The listing builds one solid part. Answer for the finished solid, in the listing's coordinates (mm). A direction names the side the tool comes from. Coordinates: 2 decimals unless noted, no trailing zeros. Write each loop counter-clockwise with the first axis right and the second up, starting at its lowest first coordinate (ties: lowest second). Pieces come first, ordered by that corner, then holes.
(1) Straight lines are drawn through the part: line 1 (Z direction, x = -22, y = 50) (3 decimals); line 2 (X direction, y = 52.5, z = 26) (3 decimals); line 3 (Z direction, x = -67, y = 2) (3 decimals). For each, find the intervals that lie inside material, in ascending order.
(2) The part is cut by section B-B on x = 67.31. Determine the outline of the cut face in (y, z) (1 decimal), plus the area to 3 significant figures.
(3) The part is cut by section D-D on x = 32. Determine the outline of the cut face in (y, z) (3 decimals), plus the area to 3 significant figures.
(4) Given P1, Ø13.5, axis at x = -72, z = 75.5, coming from the +Y side (3 decimals); P2, Ø3, axis at x = -9, y = 51, coming from the -Z side; P3, Ø7.5, axis at x = 67.31, z = -79.375, coming from the -Y side; P4, Ø2, axis at x = -41, z = -2.5, coming from the -Y side (3 decimals), each flat-ended and moving along its own axis, determine where each tip first touches the part or whether it passes through.
(5) Which of the six approach directions +Z, -Z, +X, -X, +Y, -Y give full straight-line access (tool end or side, diameter ignored) to faces 1 (the flat face through (65, 3.175, -84)), 2 (the flat face through (-83.185, 40, 1)), 3 (the flat face through (48.26, 7, -79)), 4 (the flat face through (51.435, 12, 73))?
(6) The part is cut by section C-C on z = 3. Determine the outline of the cut face in (x, y) (3 decimals), plus the area to 3 significant figures.
(7) For a pull along X with two mould halves and no side action, classify faces 5 (the flat face through (84.813, 13.568, 83.599)), 6 (the flat face through (-65, 3.175, -84)) as +X half, -X half, draft (parallel to the pull), parting line (faces both ways), or undercut.
(8) The part is cut by section A-A on y = 31. Determine the outline of the cut face in (x, z) (3 decimals).
from build123d import *

# Parameters (mm, degrees)
SKETCH1_W                    = 172.72
SKETCH1_H                    = 127
BOSS_EXTRUDE1_DEPTH          = 83.82
SHELL1_T                     = -3.175
SKETCH6_W                    = 38.1
SKETCH6_H                    = 38.1
BOSS_EXTRUDE4_DEPTH          = 3.175
BOSS_EXTRUDE5_DEPTH          = 3.175
MIRROR5_COPY_1_DEPTH         = 3.175
MIRROR6_COPY_1_DEPTH         = 3.175
MIRROR6_COPY_2_SKETCH_W      = 38.1
MIRROR6_COPY_2_SKETCH_H      = 38.1
MIRROR6_COPY_2_DEPTH         = 3.175
MIRROR6_COPY_3_DEPTH         = 3.175
MIRROR6_COPY_4_DEPTH         = 3.175
FILLET3_R                    = 2.54
F_3_8_0_375_DIAMETER_HOLE1_D = 9.525
MIRROR8_COPY_1_D             = 9.525
FILLET4_R                    = 3.175


with BuildPart() as part:
    # Sketch1 → Boss-Extrude1 (new body)
    with BuildSketch(Plane(origin=(0, 0, 0), x_dir=(1, 0, 0), z_dir=(0, 1, 0))):
        Rectangle(SKETCH1_W, SKETCH1_H)
    extrude(amount=BOSS_EXTRUDE1_DEPTH)

    # Shell1
    shell1_openings = [part.faces().sort_by_distance(p)[0] for p in [
        (0, 0, 0),
    ]]
    offset(amount=SHELL1_T, openings=shell1_openings, kind=Kind.INTERSECTION)

    # Sketch6 → Boss-Extrude4 (add)
    with BuildSketch(Plane.XZ):
        with Locations((-67.31, 82.55)):
            Rectangle(SKETCH6_W, SKETCH6_H)
    boss_extrude4 = extrude(amount=-BOSS_EXTRUDE4_DEPTH)

    # Sketch7 → Boss-Extrude5 (add)
    with BuildSketch(Plane.ZY.offset(86.36)):
        Polygon((101.6, 3.175), (63.5, 25.172045256), (63.5, 3.175), align=None)
    boss_extrude5 = extrude(amount=-BOSS_EXTRUDE5_DEPTH)

    # Mirror4: Boss-Extrude5 across plane
    add(boss_extrude5.mirror(Plane.ZY.offset(67.31)))

    # Mirror5: Boss-Extrude4, Boss-Extrude5 across plane
    add(boss_extrude4.mirror(Plane.XY))
    add(boss_extrude5.mirror(Plane.XY))

    # Mirror5 copy 1 sketch → Mirror5 copy 1 (add)
    with BuildSketch(Plane(origin=(-48.26, 0, 0), x_dir=(0, 0, -1), z_dir=(1, 0, 0))):
        Polygon((101.6, 3.175), (63.5, 25.172045256), (63.5, 3.175), align=None)
    extrude(amount=-MIRROR5_COPY_1_DEPTH)

    # Mirror6: Boss-Extrude4, Boss-Extrude5 across plane
    add(boss_extrude4.mirror(Plane(origin=(0, 0, 0), x_dir=(0, 0, 1), z_dir=(1, 0, 0))))
    add(boss_extrude5.mirror(Plane(origin=(0, 0, 0), x_dir=(0, 0, 1), z_dir=(1, 0, 0))))

    # Mirror6 copy 1 sketch → Mirror6 copy 1 (add)
    with BuildSketch(Plane.ZY.offset(-48.26)):
        Polygon((101.6, 3.175), (63.5, 25.172045256), (63.5, 3.175), align=None)
    extrude(amount=-MIRROR6_COPY_1_DEPTH)

    # Mirror6 copy 2 sketch → Mirror6 copy 2 (add)
    with BuildSketch(Plane(origin=(0, 0, 0), x_dir=(-1, 0, 0), z_dir=(0, -1, 0))):
        with Locations((-67.31, 82.55)):
            Rectangle(MIRROR6_COPY_2_SKETCH_W, MIRROR6_COPY_2_SKETCH_H)
    extrude(amount=-MIRROR6_COPY_2_DEPTH)

    # Mirror6 copy 3 sketch → Mirror6 copy 3 (add)
    with BuildSketch(Plane(origin=(86.36, 0, 0), x_dir=(0, 0, -1), z_dir=(1, 0, 0))):
        Polygon((101.6, 3.175), (63.5, 25.172045256), (63.5, 3.175), align=None)
    extrude(amount=-MIRROR6_COPY_3_DEPTH)

    # Mirror6 copy 4 sketch → Mirror6 copy 4 (add)
    with BuildSketch(Plane(origin=(48.26, 0, 0), x_dir=(0, 0, -1), z_dir=(-1, 0, 0))):
        Polygon((101.6, -3.175), (63.5, -25.172045256), (63.5, -3.175), align=None)
    extrude(amount=-MIRROR6_COPY_4_DEPTH)

    # Fillet3
    fillet3_edges = [part.edges().sort_by_distance(p)[0] for p in [
        (51.435, 3.175, -82.55),
        (67.31, 3.175, -63.5),
        (83.185, 3.175, -82.55),
        (51.435, 3.175, 82.55),
        (67.31, 3.175, 63.5),
        (83.185, 3.175, 82.55),
        (-67.31, 3.175, 63.5),
        (-83.185, 3.175, 82.55),
        (-51.435, 3.175, 82.55),
        (-51.435, 3.175, -82.55),
        (-67.31, 3.175, -63.5),
        (-83.185, 3.175, -82.55),
    ]]
    fillet(fillet3_edges, radius=FILLET3_R)

    # 3/8 (0.375) Diameter Hole1 (through all)
    with Locations(Plane(origin=(0, 3.175, 0), x_dir=(1, 0, 0), z_dir=(0, 1, 0))):
        with Locations((-67.31, -79.375)):
            f_3_8_0_375_diameter_hole1 = Hole(F_3_8_0_375_DIAMETER_HOLE1_D / 2)

    # Mirror7: 3/8 (0.375) Diameter Hole1 across plane
    add(f_3_8_0_375_diameter_hole1.mirror(Plane.XY), mode=Mode.SUBTRACT)

    # Mirror8: 3/8 (0.375) Diameter Hole1 across plane
    add(f_3_8_0_375_diameter_hole1.mirror(Plane(origin=(0, 0, 0), x_dir=(0, 0, 1), z_dir=(1, 0, 0))), mode=Mode.SUBTRACT)

    # Mirror8 copy 1 (through all)
    with Locations(Plane(origin=(0, 3.175, 0), x_dir=(-1, 0, 0), z_dir=(0, 1, 0))):
        with Locations((-67.31, -79.375)):
            Hole(MIRROR8_COPY_1_D / 2)

    # Fillet4
    fillet4_edges = [part.edges().sort_by_distance(p)[0] for p in [
        (49.8475, 25.172045256, -63.5),
        (84.7725, 25.172045256, -63.5),
        (49.8475, 25.172045256, 63.5),
        (84.7725, 25.172045256, 63.5),
        (-84.7725, 25.172045256, 63.5),
        (-49.8475, 25.172045256, 63.5),
        (-49.8475, 25.172045256, -63.5),
        (-84.7725, 25.172045256, -63.5),
    ]]
    fillet(fillet4_edges, radius=FILLET4_R)


solid = part.part
Model answer:
1. line 1: z = -63.5 to -60.325, 60.325 to 63.5
1. line 2: x = -86.36 to -83.185, 83.185 to 86.36
1. line 3: z = -101.6 to -84.127, -74.623 to -60.325, 60.325 to 74.623, 84.127 to 101.6
2. outline: (0, -101.6) - (3.2, -101.6) - (3.2, -84.1) - (0, -84.1) - close; (0, -74.6) - (3.2, -74.6) - (3.2, -66) arc R2.5 cw to (5.7, -63.5) - (83.8, -63.5) - (83.8, 63.5) - (5.7, 63.5) arc R2.5 cw to (3.2, 66) - (3.2, 74.6) - (0, 74.6) - (0, 60.3) - (80.6, 60.3) - (80.6, -60.3) - (0, -60.3) - close; (0, 84.1) - (3.2, 84.1) - (3.2, 101.6) - (0, 101.6) - close
2. area: 1,100 mm2
3. outline: (0, -63.5) - (83.82, -63.5) - (83.82, 63.5) - (0, 63.5) - (0, 60.325) - (80.645, 60.325) - (80.645, -60.325) - (0, -60.325) - close
3. area: 915 mm2
4. P1: stops at y = 3.175
4. P2: stops at z = -63.5
4. P3: passes through
4. P4: stops at y = 80.645
5. face 1: -Z, +Y
5. face 2: -Y
5. face 3: -Z, +Y, -Y
5. face 4: +Z, +Y
6. outline: (-86.36, 0) - (-83.185, 0) - (-83.185, 80.645) - (83.185, 80.645) - (83.185, 0) - (86.36, 0) - (86.36, 83.82) - (-86.36, 83.82) - close
6. area: 1,060 mm2
7. face 5: draft
7. face 6: undercut
8. outline: (-86.36, -63.5) - (86.36, -63.5) - (86.36, 63.5) - (-86.36, 63.5) - close; hole (-83.185, -60.325) - (83.185, -60.325) - (83.185, 60.325) - (-83.185, 60.325) - close
